from build123d import *

# Parameters (mm, degrees)
F2_R       = 14.09
F0_R       = 14.72
F3_FACE_R  = 14.09
F7_R       = 3.265
F4_R       = 13.72
F5_R       = 13.09
F10_FACE_R = 13.09
F11_R      = 2.6


with BuildPart() as f3:
    # F2 (on offset) → F3 section 0
    with BuildSketch(Plane.XZ.offset(-98)):
        Circle(F2_R)
    # F0 (on Front) → F3 section 1
    with BuildSketch(Plane.XZ):
        Circle(F0_R)
    loft()

    # F3_face (on face) → F9 section 0
    with BuildSketch(Plane(origin=(0, 98, 0), x_dir=(-1, 0, 0), z_dir=(0, 1, 0))):
        Circle(F3_FACE_R)
    # F7 (on offset) → F9 section 1
    with BuildSketch(Plane.XZ.offset(-114.3)):
        Circle(F7_R)
    loft()

    # F4 (on Front) → F10 section 0
    with BuildSketch(Plane.XZ):
        Circle(F4_R)
    # F5 (on offset) → F10 section 1
    with BuildSketch(Plane.XZ.offset(-98)):
        Circle(F5_R)
    loft(mode=Mode.SUBTRACT)

    # F10_face (on face) → F12 section 0
    with BuildSketch(Plane.XZ.offset(-98)):
        Circle(F10_FACE_R)
    # F11 (on offset) → F12 section 1
    with BuildSketch(Plane.XZ.offset(-113.3)):
        Circle(F11_R)
    loft(mode=Mode.SUBTRACT)


solid = f3.part
Build history of the part. All positions in model axes, mm. A direction names the side the tool comes from. Coordinates: 2 decimals unless noted, no trailing zeros. Write each loop counter-clockwise with the first axis right and the second up, starting at its lowest first coordinate (ties: lowest second). Pieces come first, ordered by that corner, then holes.
(1) Drill centre lines: line 1 (Z direction, x = 10, y = 23); line 2 (X direction, y = 19.5, z = -3.75); line 3 (Z direction, x = -8.5, y = 92). Where is each one in solid material? Low to high.
(2) 3-axis set-ups, long thin cutter, end or side, ignore diameter. For faces 4 (the conical face through (12.78, 49.69, 4.03)), 5 (the conical face through (-3.124, 48.314, -14.067)), 6 (the flat face through (0, 114.3, 0)): which of +Z, -Z, +X, -X, +Y, -Y reach the whole face in a straight line?
(3) Pin check, flat tips, straight feed: pin 1 Ø3 at (x, z) = (-0.5, -9.5) entering from +Y; pin 2 Ø5 at (x, y) = (5.5, 39) entering from -Z; pin 3 Ø8 at (x, y) = (-10.5, 92.5) entering from +Z. Stop position of each tip, or through.
(4) Cut at A-A on y = 105.5. List the corners of the cut face in (x, z).
(5) Mould opens along Z. For faces 1 (the flat face through (0, 113.3, 0)), 2 (the flat face through (-12, 0, 7)), 3 (the conical face through (-2.859, 109.886, -5.497)) say: pulls with the +Z half, pulls with the -Z half, needs draft (parallel to the pull), parting line crosses it, or undercut.
(6) Cut at B-B on y = 84. List the corners of the cut face in (x, z), and give its area (3 significant figures).
Working result:
1. line 1: z = -10.6 to -9.18, 9.18 to 10.6
1. line 2: x = -14.1 to -13.07, 13.07 to 14.1
1. line 3: z = -11.29 to -10.01, 10.01 to 11.29
2. face 4: -Y
2. face 5: +Y
2. face 6: +Z, -Z, +X, -X, +Y
3. pin 1: stops at y = 107.15
3. pin 2: stops at z = -14.16
3. pin 3: stops at z = 12.54
4. outline: circle Ø18.22 at (0, 0); hole circle Ø15.9 at (0, 0)
5. face 1: undercut
5. face 2: needs draft
5. face 3: parting line crosses it
6. outline: circle Ø28.36 at (0, 0); hole circle Ø26.36 at (0, 0)
6. area: 86.0 mm2
